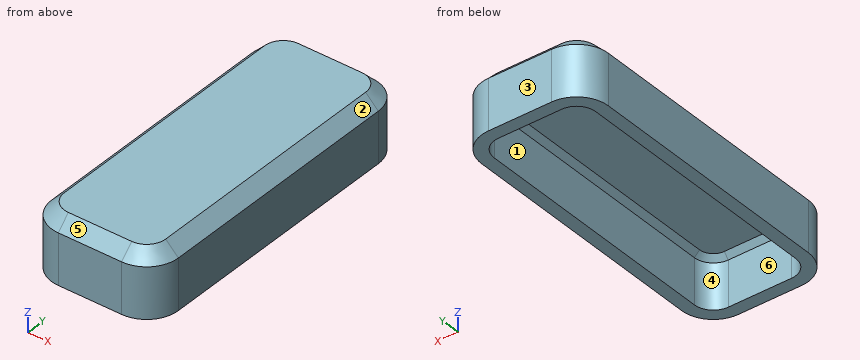
from build123d import *

# Parameters (mm, degrees)
F0_W     = 50.8
F0_H     = 25.4
F1_DEPTH = 127
F2_R     = 12.7
F3_SIZE  = 5.08
F4_T     = -5.08


with BuildPart() as f1:
    # F0 (on Front) → F1 (new body)
    with BuildSketch(Plane.XZ):
        with Locations((25.4, 12.7)):
            Rectangle(F0_W, F0_H)
    extrude(amount=-F1_DEPTH)

    # F2
    f2_edges = [f1.edges().sort_by_distance(p)[0] for p in [
        (0, 0, 12.7),
        (50.8, 0, 12.7),
        (50.8, 127, 12.7),
        (0, 127, 12.7),
    ]]
    fillet(f2_edges, radius=F2_R)

    # F3
    f3_edges = [f1.edges().sort_by_distance(p)[0] for p in [
        (50.8, 63.5, 25.4),
    ]]
    chamfer(f3_edges, length=F3_SIZE)

    # F4
    f4_openings = [f1.faces().sort_by_distance(p)[0] for p in [
        (25.4, 63.5, 0),
    ]]
    offset(amount=F4_T, openings=f4_openings)


solid = f1.part
Read the model definition and answer for the solid it produces. Units are mm, in the model's axes. Face numbers are marked on the shaded views. A direction names the side the tool comes from. Round coordinates to 2 decimals unless told otherwise and drop trailing zeros. Loops run counter-clockwise (first coordinate to the right, second up) from the corner with the lowest first, then second, coordinate; pieces in that order, holes last.
Q1. Section D-D on z = 23 is taken. Write down the section's boundary in (x, y).
Q2. Consider probe 1 along X at (y, z) = (40.5, 14); probe 2 along Y at (x, z) = (33, 16.75); probe 3 along Z at (x, y) = (32, 45). Determine where each line is inside the solid, lowest interval first.
Q3. Each of these flat-tipped pins is pushed along its axis until it touches: pin 1 (11 mm diameter, centred on x = 26.5, y = 42.5, fed in from -Z); pin 2 (1 mm diameter, centred on y = 17, z = 22, fed in from -X). Where does it stop, or does it pass through?
Q4. Section A-A on y = 66 is taken. Write down the section's boundary in (x, z), and give its area (3 significant figures).
Q5. Determine the mould class of the marked faces 1, 2, 3 and 4 for opening direction Y: released by +Y, released by -Y, zero draft, split by the parting line, or undercut.
Q6. Section B-B on x = 19 is taken. Write down the section's boundary in (y, z).
Q7. Which of the six approach directions +Z, -Z, +X, -X, +Y, -Y give full straight-line access (tool end or side, diameter ignored) to the marked faces 5 and 6?
Q8. Section C-C on z = 8 is taken. Write down the section's boundary in (x, y).
Output:
1. outline: (2.68, 12.7) arc R10.02 ccw to (12.7, 2.68) - (38.1, 2.68) arc R10.02 ccw to (48.12, 12.7) - (48.12, 114.3) arc R10.02 ccw to (38.1, 124.32) - (12.7, 124.32) arc R10.02 ccw to (2.68, 114.3) - close
2. probe 1: x = 0 to 5.08, 45.72 to 50.8
2. probe 2: y = 0 to 5.08, 121.92 to 127
2. probe 3: z = 20.32 to 25.4
3. pin 1: stops at z = 20.32
3. pin 2: stops at x = 1.18
4. outline: (0, 0) - (5.08, 0) - (5.08, 18.22) - (7.18, 20.32) - (43.62, 20.32) - (45.72, 18.22) - (45.72, 0) - (50.8, 0) - (50.8, 20.32) - (45.72, 25.4) - (5.08, 25.4) - (0, 20.32) - close
4. area: 443 mm2
5. face 1: undercut
5. face 2: zero draft
5. face 3: released by +Y
5. face 4: undercut
6. outline: (0, 0) - (5.08, 0) - (5.08, 18.22) - (7.18, 20.32) - (119.82, 20.32) - (121.92, 18.22) - (121.92, 0) - (127, 0) - (127, 20.32) - (121.92, 25.4) - (5.08, 25.4) - (0, 20.32) - close
7. face 5: +Z, +X, -X, -Y
7. face 6: -Z
8. outline: (0, 12.7) arc R12.7 ccw to (12.7, 0) - (38.1, 0) arc R12.7 ccw to (50.8, 12.7) - (50.8, 114.3) arc R12.7 ccw to (38.1, 127) - (12.7, 127) arc R12.7 ccw to (0, 114.3) - close; hole (5.08, 12.7) arc R7.62 ccw to (12.7, 5.08) - (38.1, 5.08) arc R7.62 ccw to (45.72, 12.7) - (45.72, 114.3) arc R7.62 ccw to (38.1, 121.92) - (12.7, 121.92) arc R7.62 ccw to (5.08, 114.3) - close
